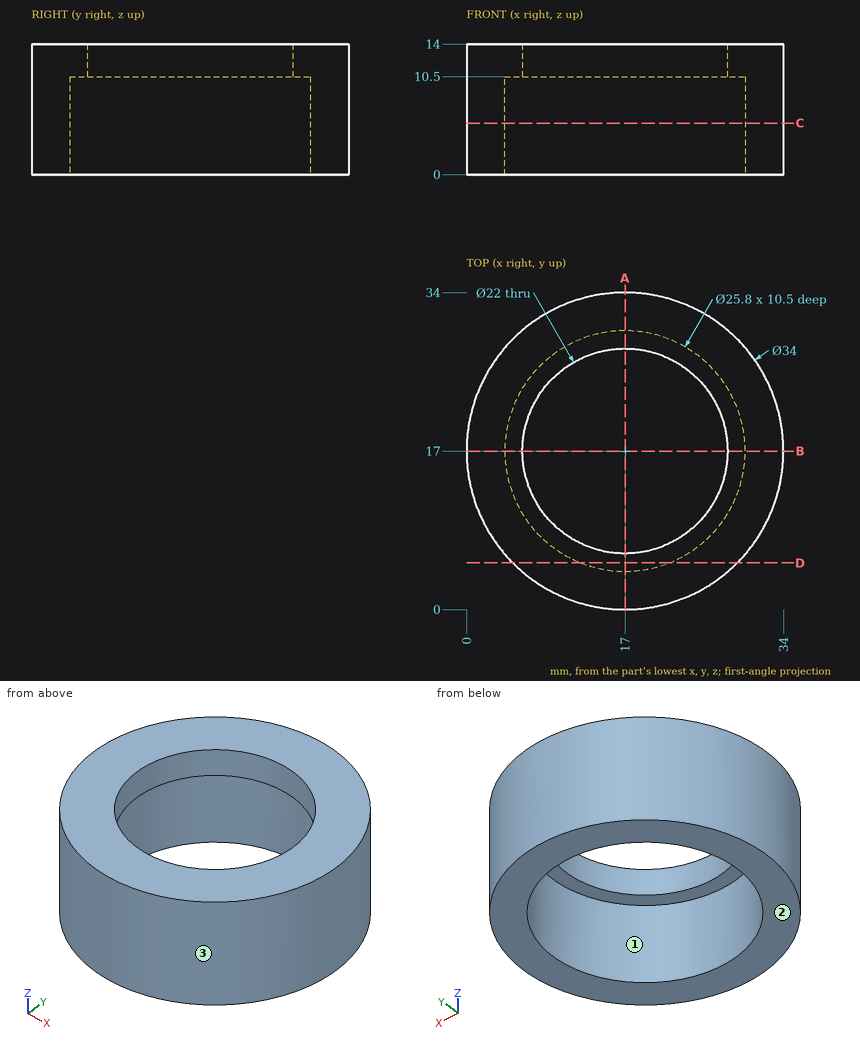
Geometry check sheet. Reference: drawing and pictorial views, mm from the part's lowest x, y, z. Coordinates: 2 decimals unless noted, no trailing zeros. Write each loop counter-clockwise with the first axis right and the second up, starting at its lowest first coordinate (ties: lowest second). Pieces come first, ordered by that corner, then holes. Notation, with made-up numbers: M 48.5,75 L 52.5,75 A27 ccw 52.5,93 Z; hole C 68.25,-28 d1. An arc over 180 degrees is marked long. Write item = value, one per line. Start each with the question number.
1. Mould release check, pull along Y, two halves, no side actions. Record for the marked faces 1, 2 and 3: pulls with the +Y half, pulls with the -Y half, needs draft (parallel to the pull), parting line crosses it, or undercut.
2. Thickness scan on probe 1 along Y at (x, z) = (17, 13.2); probe 2 along Y at (x, z) = (17, 5.5); probe 3 along X at (y, z) = (17.5, 9.25). Record the ranges inside material, lowest first.
3. Sectioned sample at A-A (x = 17). Record the cut outline in (y, z), then the cut area to 3 significant figures.
4. Go/stop test with flat-tipped pins: pin 1 (1.5 mm diameter, centred on x = 16, y = 6.5, fed in from +Z); pin 2 (8 mm diameter, centred on x = 6, z = 11, fed in from +Y); pin 3 (3 mm diameter, centred on x = 9.5, z = 7.5, fed in from +Y); pin 4 (8 mm diameter, centred on y = 6, z = 3.5, fed in from +X). Record where each tip stops, or that it passes through.
5. Sectioned sample at C-C (z = 5.5). Record the cut outline in (x, y).
6. Sectioned sample at D-D (y = 5). Record the cut outline in (x, z).
The answers:
q1.face_1 = undercut
q1.face_2 = needs draft
q1.face_3 = parting line crosses it
q2.probe_1 = 0 to 6, 28 to 34
q2.probe_2 = 0 to 4.1, 29.9 to 34
q2.probe_3 = 0.01 to 4.11, 29.89 to 33.99
q3.outline = M 0,0 L 4.1,0 L 4.1,10.5 L 6,10.5 L 6,14 L 0,14 Z; M 28,10.5 L 29.9,10.5 L 29.9,0 L 34,0 L 34,14 L 28,14 Z
q3.area = 128 mm²
q4.pin_1 = 14
q4.pin_2 = 32.49
q4.pin_3 = 32.91
q4.pin_4 = 32.49
q5.outline = C 17,17 d34; hole C 17,17 d25.8
q6.outline = M 4.96,0 L 12.27,0 L 12.27,10.5 L 21.73,10.5 L 21.73,0 L 29.04,0 L 29.04,14 L 4.96,14 Z
